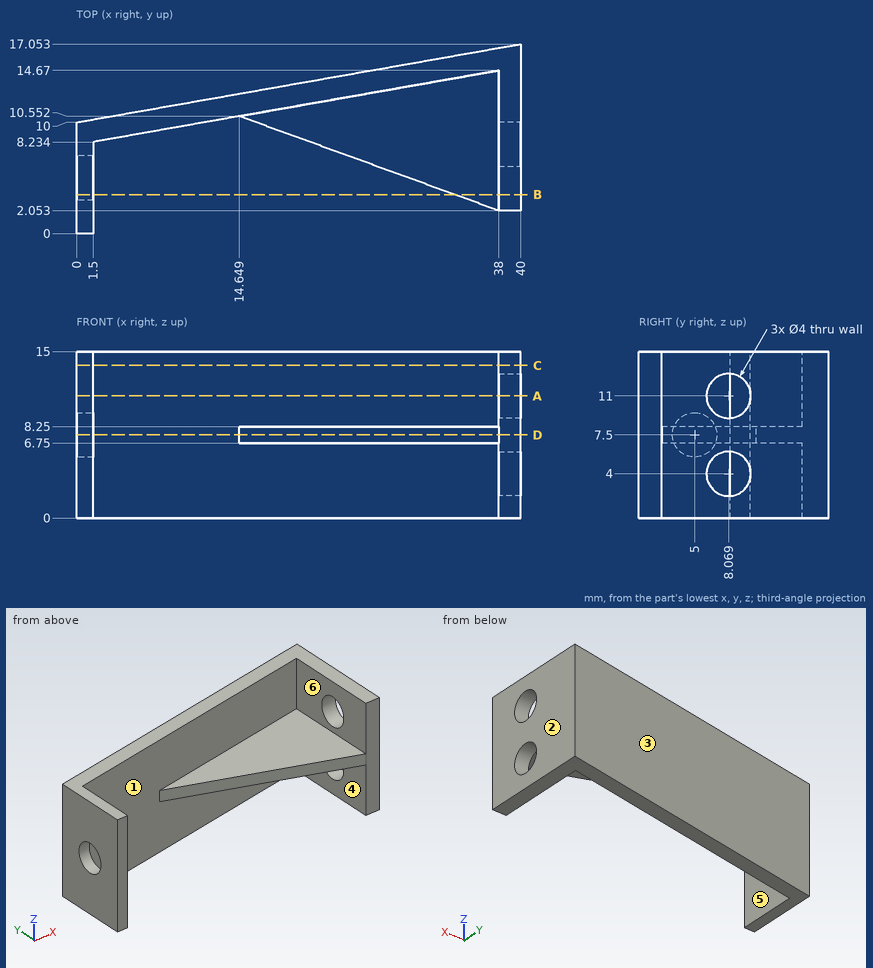
Source: three-view drawing plus pictorial views. Frame: mm from the lowest corner of the part. A direction names the side the tool comes from. Round coordinates to 2 decimals unless told otherwise and drop trailing zeros. Loops run counter-clockwise (first coordinate to the right, second up) from the corner with the lowest first, then second, coordinate; pieces in that order, holes last. Notation, with made-up numbers: M 73.25,-16.5 L 129.25,-16.5 A12 cw 129.25,-3.5 Z; hole C 81.25,55 d8. An arc over 180 degrees is marked long. Put each result on its own line as item: value.
(1) Pull-direction query (X, two-part tool) for the marked faces 1, 2 and 3; classes: released by +X, released by -X, zero draft, split by the parting line, or undercut.
Solutions:
face 1: undercut
face 2: released by +X
face 3: released by -X
(2) First-contact query: pin 1 (1.5 mm diameter, centred on x = 30, z = 11, fed in from +Y); pin 2 (2 mm diameter, centred on x = 38.5, z = 4.5, fed in from -Y); pin 3 (8 mm diameter, centred on x = 9.5, z = 1.5, fed in from +Y). Flat tips, straight axial feed; report the tip coordinate or a pass-through.
Solutions:
pin 1: y = 15.42
pin 2: y = 2.05
pin 3: y = 12.38
(3) Section D-D, the plane z = 7.5. Return loops of the section in (x, y), and give its area (3 significant figures).
Solutions:
outline: M 0,0 L 1.5,0 L 1.5,3 L 0,3 Z; M 0,7 L 1.5,7 L 1.5,8.23 L 14.65,10.55 L 38,2.05 L 40,2.05 L 40,17.05 L 0,10 Z
area: 260 mm²
(4) Access query for the marked faces 4, 5 and 6. Directions: +Z, -Z, +X, -X, +Y, -Y. A direction counts if a zero-diameter tool reaches every point of the face in a straight line with its end or side. Return the directions, or none.
Solutions:
face 4: -Z, -Y
face 5: +Z, -Z, -Y
face 6: +Z, -Y
(5) Section A-A, the plane z = 11. Return loops of the section in (x, y).
Solutions:
outline: M 0,0 L 1.5,0 L 1.5,8.23 L 38,14.67 L 38,10.07 L 40,10.07 L 40,17.05 L 0,10 Z; M 38,2.05 L 40,2.05 L 40,6.07 L 38,6.07 Z
(6) Section C-C, the plane z = 13.75. Return loops of the section in (x, y).
Solutions:
outline: M 0,0 L 1.5,0 L 1.5,8.23 L 38,14.67 L 38,2.05 L 40,2.05 L 40,17.05 L 0,10 Z
(7) Section B-B, the plane y = 3.5. State how many separate pieces and enclosed holes the cut face has.
Solutions:
separate pieces: 3
enclosed holes: 0
(8) Ray query, line 1 (X direction, y = 5.75, z = 11); line 2 (X direction, y = 8, z = 12.5); line 3 (Y direction, x = 0.7, z = 7.5). Return the intervals inside material, ascending. Write a range as [from, to].
Solutions:
line 1: [0, 1.5], [38, 40]
line 2: [0, 1.5]
line 3: [0, 3], [7, 10.12]
